```python
from build123d import *

# Parameters (mm, degrees)
F1_DEPTH = 3
F2_R     = 1.33
F3_DEPTH = 3.001


with BuildPart() as f1:
    # F0 (on Front) → F1 (new body)
    with BuildSketch(Plane.XZ):
        with BuildLine():
            ThreePointArc((-19.35648, 34.085312), (-21.41906, 33.046163), (-22.25, 30.891259))
            Line((-22.25, 30.891259), (-22.25, -30.860331))
            ThreePointArc((-22.25, -30.860331), (-21.32844, -33.100719), (-19.097213, -34.04424))
            Line((-19.097213, -34.04424), (-15.3672, -34.04424))
            ThreePointArc((-15.3672, -34.04424), (-13.279512, -33.719597), (-11.44242, -32.676084))
            Line((-11.44242, -32.676084), (-9.386582, -31.040758))
            ThreePointArc((-9.386582, -31.040758), (-7.333283, -29.983659), (-5.04129, -29.700344))
            Line((-5.04129, -29.700344), (0, -29.700344))
            Line((0, -29.700344), (5.04129, -29.700344))
            ThreePointArc((5.04129, -29.700344), (7.333283, -29.983659), (9.386582, -31.040758))
            Line((9.386582, -31.040758), (11.44242, -32.676084))
            ThreePointArc((11.44242, -32.676084), (13.279512, -33.719597), (15.3672, -34.04424))
            Line((15.3672, -34.04424), (19.097213, -34.04424))
            ThreePointArc((19.097213, -34.04424), (21.32844, -33.100719), (22.25, -30.860331))
            Line((22.25, -30.860331), (22.25, 30.891259))
            ThreePointArc((22.25, 30.891259), (21.41906, 33.046163), (19.35648, 34.085312))
            ThreePointArc((19.35648, 34.085312), (16.119272, 33.397026), (13.494445, 31.381204))
            ThreePointArc((13.494445, 31.381204), (11.432837, 30.084307), (9.027799, 29.699656))
            Line((9.027799, 29.699656), (0, 29.699656))
            Line((0, 29.699656), (-9.027799, 29.699656))
            ThreePointArc((-9.027799, 29.699656), (-11.432837, 30.084307), (-13.494445, 31.381204))
            ThreePointArc((-13.494445, 31.381204), (-16.119272, 33.397026), (-19.35648, 34.085312))
        make_face()
    extrude(amount=F1_DEPTH)

    # F2 (on face) → F3 (cut, through all)
    with BuildSketch(Plane.XZ.offset(3)):
        with Locations((-19.175, 31.125)):
            Circle(F2_R)
        with Locations((19.175, 31.125)):
            Circle(F2_R)
        with Locations((19.175, -31.125)):
            Circle(F2_R)
        with Locations((-19.175, -31.125)):
            Circle(F2_R)
    extrude(amount=-F3_DEPTH, mode=Mode.SUBTRACT)


solid = f1.part
```
Input: part model. Units: mm. Frame: model coordinates. A direction names the side the tool comes from. Round coordinates to 2 decimals unless told otherwise and drop trailing zeros. Write each loop counter-clockwise with the first axis right and the second up, starting at its lowest first coordinate (ties: lowest second). Pieces come first, ordered by that corner, then holes. Notation, with made-up numbers: M 32,59.25 L 74,59.25 A18 ccw 74,71.25 Z; hole C -18,-16 d5. An arc over 180 degrees is marked long. Write each question's results on one line, items separated by ' | '.
Q1. Draft query along Z for faces 4 (the face through (0, -1, 29.7)), 5 (the face through (-17.946, -1.521, -31.634)), 6 (the face through (0, -1, -29.7)). Return one class per face: released by +Z, released by -Z, zero draft, split by the parting line, or undercut.
Results:
face 4: released by +Z | face 5: undercut | face 6: released by -Z
Q2. Line query: line 1 along X through (y, z) = (-0.7, 31.5); line 2 along Z through (x, y) = (-4, -1.85); line 3 along Z through (x, y) = (-12, -0.3). Output: solid intervals per line, ascending.
Results:
line 1: x = -22.19 to -20.45, -17.9 to -13.6, 13.6 to 17.9, 20.45 to 22.19 | line 2: z = -29.7 to 29.7 | line 3: z = -33.09 to 30.33
Q3. Pin query (flat end, axial travel): P1, Ø4.5, axis at x = -19.175, z = 31.125, coming from the -Y side; P2, Ø1.6, axis at x = 19.175, z = 31.125, coming from the +Y side; P3, Ø0.9, axis at x = -2.5, y = -1, coming from the -Z side; P4, Ø0.9, axis at x = 18, y = -2, coming from the -Z side. Return the tip coordinate at first contact, or that it passes through.
Results:
P1: stops at y = -3 | P2: passes through | P3: stops at z = -29.7 | P4: stops at z = -34.04
Q4. Section query A-A (y = -0.85). State how many separate pieces and enclosed holes the cut face has, and give its area (3 significant figures).
Results:
separate pieces: 1 | enclosed holes: 4 | area: 2,790 mm^2
Q5. Access query for faces 1 (the face through (16.162, -1.479, 33.416)), 2 (the face through (-10.43, -1.48, -31.87)), 3 (the face through (22.25, -1, 0)). Directions: +Z, -Z, +X, -X, +Y, -Y. A direction counts if a zero-diameter tool reaches every point of the face in a straight line with its end or side. Return the directions, or none.
Results:
face 1: +Z, +Y, -Y | face 2: -Z, +Y, -Y | face 3: +Z, -Z, +X, +Y, -Y
Q6. Section query B-B (x = 3.5). Return loops of the section in (y, z), and give its area (3 significant figures).
Results:
outline: M -3,-29.7 L 0,-29.7 L 0,29.7 L -3,29.7 Z | area: 178 mm^2
